Geometry check sheet. Reference: drawing and pictorial views, mm from the part's lowest x, y, z. A direction names the side the tool comes from. Give positions to 0.01 mm unless a question says otherwise; leave off trailing zeros. Loops run counter-clockwise (first coordinate to the right, second up) from the corner with the lowest first, then second, coordinate; pieces in that order, holes last. Notation, with made-up numbers: (14.25, 5) -> (62.25, 5) arc R8 ccw to (62.25, 13) -> close; hole circle Ø9 at (-36.5, 43). An arc over 180 degrees is marked (long way). One line per item, written item: value. Start each with the question number.
(1) Sectioned sample at C-C, the plane z = 3. Record the cut outline in (x, y).
(2) Draft check along X on the marked faces 1, 2 and 3. Enter one of: pulls with the +X half, pulls with the -X half, needs draft (parallel to the pull), parting line crosses it, or undercut.
(3) Sectioned sample at D-D, the plane x = 11.5. Record the cut outline in (y, z), then the cut area to 3 significant figures.
(4) Scan lines: line 1 along X through (y, z) = (1.9, 3); line 2 along Z through (x, y) = (5, 2.7); line 3 along X through (y, z) = (15, 26.75). Record each from-to range of solid material in increasing order. Write a range as from..to.
(5) Tool access check on the marked faces 4 and 5. Record the directions out of +Z, -Z, +X, -X, +Y, -Y that give a thin tool (end or side, any length) a straight path to the whole face; none if there is none.
(6) Gauge pin test, flat ends, axial feed: pin 1 Ø16 at (x, z) = (27.5, 9.5) entering from +Y; pin 2 Ø5 at (x, z) = (5.5, 20.5) entering from +Y. Record the tip position at first contact, or that the pin passes through.
(7) Sectioned sample at B-B, the plane x = 4. Record the cut outline in (y, z), then the cut area to 3 significant figures.
(8) Sectioned sample at A-A, the plane y = 20. Record the cut outline in (x, z) (3 decimals), then the cut area to 3 significant figures.
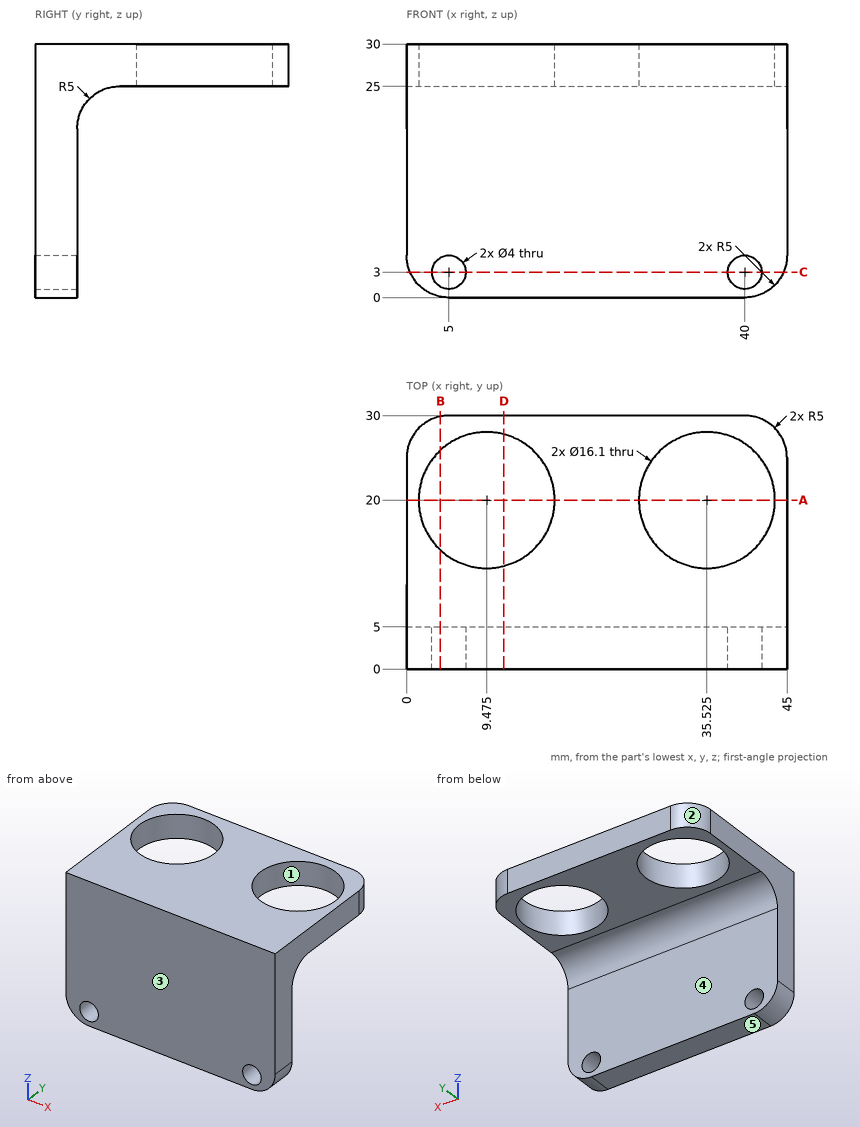
Calculated:
1. outline: (0.42, 0) -> (3, 0) -> (3, 5) -> (0.42, 5) -> close; (7, 0) -> (38, 0) -> (38, 5) -> (7, 5) -> close; (42, 0) -> (44.58, 0) -> (44.58, 5) -> (42, 5) -> close
2. face 1: undercut
2. face 2: pulls with the -X half
2. face 3: needs draft
3. outline: (0, 0) -> (5, 0) -> (5, 20) arc R5 cw to (10, 25) -> (12.21, 25) -> (12.21, 30) -> (0, 30) -> close; (27.79, 25) -> (30, 25) -> (30, 30) -> (27.79, 30) -> close
3. area: 202 mm2
4. line 1: x = 0.42..3, 7..38, 42..44.58
4. line 2: z = 0..1, 5..30
4. line 3: x = 0..3.17, 15.78..29.22, 41.83..45
5. face 4: -Z, +X, -X, +Y
5. face 5: -Z, +X, -X, +Y, -Y
6. pin 1: stops at y = 5
6. pin 2: stops at y = 6
7. outline: (0, 0.1) -> (5, 0.1) -> (5, 1.27) -> (0, 1.27) -> close; (0, 4.73) -> (5, 4.73) -> (5, 20) arc R5 cw to (10, 25) -> (14.1, 25) -> (14.1, 30) -> (0, 30) -> close; (25.9, 25) -> (29.9, 25) -> (29.9, 30) -> (25.9, 30) -> close
7. area: 203 mm2
8. outline: (0, 25) -> (1.425, 25) -> (1.425, 30) -> (0, 30) -> close; (17.525, 25) -> (27.475, 25) -> (27.475, 30) -> (17.525, 30) -> close; (43.575, 25) -> (45, 25) -> (45, 30) -> (43.575, 30) -> close
8. area: 64.0 mm2
